from build123d import *

# Parameters (mm, degrees)
BOSS_EXTRUDE1_DEPTH             = 1
BOSS_EXTRUDE5_DEPTH             = 100
BOSS_EXTRUDE5_DEPTH_BACK        = 1
SKETCH2_W                       = 214
SKETCH2_H                       = 10
FILLET3_SIZE                    = 15
FILLET3_SIZE_2                  = 10
CUT_EXTRUDE2_DEPTH              = 229
SKETCH7_W                       = 64
SKETCH7_H                       = 10
CUT_EXTRUDE3_DEPTH              = 14
SKETCH11_R                      = 5
SKETCH11_R_2                    = 2.5
EXTRUDE_THIN4_DEPTH             = 23
EXTRUDE_THIN5_START             = -63.5
SKETCH11_2_R                    = 5
SKETCH11_2_R_2                  = 2.5
EXTRUDE_THIN5_DEPTH             = 23
EXTRUDE_THIN6_START             = -127
SKETCH11_3_R                    = 5
SKETCH11_3_R_2                  = 2.5
EXTRUDE_THIN6_DEPTH             = 23
SKETCH12_W                      = 210
SKETCH12_H                      = 6
CUT_EXTRUDE4_DEPTH              = 82
CUT_EXTRUDE5_DEPTH              = 180
SKETCH14_W                      = 83.209760426
SKETCH14_H                      = 10
BOSS_EXTRUDE6_DEPTH             = 2
SKETCH15_W                      = 1.646756057
SKETCH15_H                      = 0.570147936
SKETCH15_W_2                    = 1.681570062
SKETCH15_H_2                    = 0.299582691
CUT_EXTRUDE6_DEPTH              = 182
SKETCH16_W                      = 150
SKETCH16_H                      = 42
CUT_EXTRUDE7_DEPTH              = 182
BOSS_EXTRUDE7_REACH             = 107.948
BOSS_EXTRUDE7_END_RADIUS        = 5
BOSS_EXTRUDE7_START             = -10
SKETCH17_W                      = 23
SKETCH17_H                      = 5
BOSS_EXTRUDE7_DIRECTION_2_DEPTH = 1
FILLET5_SIZE                    = 10
FILLET5_SIZE_2                  = 1


with BuildPart() as part:
    # Sketch1 → Boss-Extrude1 (new body)
    with BuildSketch(Plane.XY):
        Polygon((75, 50), (75, -50), (-75, -30), (-75, 30), align=None)
    extrude(amount=BOSS_EXTRUDE1_DEPTH)

    # Sketch2 → Boss-Extrude5 (add, two sides: drawn at the far end of the back side and taken through both)
    with BuildSketch(Plane.XY.offset(1).offset(-BOSS_EXTRUDE5_DEPTH_BACK)):
        with Locations((32, 0)):
            Rectangle(SKETCH2_W, SKETCH2_H)
    extrude(amount=BOSS_EXTRUDE5_DEPTH + BOSS_EXTRUDE5_DEPTH_BACK)

    # Fillet3
    # an asymmetric fillet: 15, 10 mm, written as the material it adds along each edge
    with BuildSketch(Plane(origin=(75, -5, 1), x_dir=(0, 0, 1), z_dir=(-1, 0, 0))) as fillet3_piece_1:
        with BuildLine():
            Bezier((FILLET3_SIZE, 0), (0, 0), (0, -FILLET3_SIZE_2), weights=[1, 0.707106781, 1])
            Line((0, -FILLET3_SIZE_2), (0, 0))
            Line((0, 0), (FILLET3_SIZE, 0))
        make_face()
    extrude(amount=150)
    with BuildSketch(Plane(origin=(-75, 5, 1), x_dir=(0, 1, 0), z_dir=(1, 0, 0))) as fillet3_piece_2:
        with BuildLine():
            Bezier((FILLET3_SIZE_2, 0), (0, 0), (0, FILLET3_SIZE), weights=[1, 0.707106781, 1])
            Line((0, FILLET3_SIZE), (0, 0))
            Line((0, 0), (FILLET3_SIZE_2, 0))
        make_face()
    extrude(amount=150)

    # Sketch6 → Cut-Extrude2 (cut)
    with BuildSketch(Plane.ZY.offset(75)):
        with BuildLine():
            Line((9.5, 6.986773712), (9.5, 4.330127019))
            ThreePointArc((9.5, 4.330127019), (7, 0), (9.5, -4.330127019))
            Line((9.5, -4.330127019), (9.5, -7.297871365))
            Line((9.5, -7.297871365), (14.5, -7.297871365))
            Line((14.5, -7.297871365), (14.5, -4.330127019))
            ThreePointArc((14.5, -4.330127019), (17, 0), (14.5, 4.330127019))
            Line((14.5, 4.330127019), (14.5, 6.986773712))
            Line((14.5, 6.986773712), (9.5, 6.986773712))
        make_face()
    extrude(amount=-CUT_EXTRUDE2_DEPTH, mode=Mode.SUBTRACT)


with BuildPart() as cut_extrude2_piece_1:
    # of the separate pieces the step leaves, piece 1, a body of its own (cut_extrude2_pieces)
    add(part.part.solids().sort_by_distance((-75, 5.050125629, 14.5))[0])

    # Sketch11 → Extrude-Thin4 (add)
    with BuildSketch(Plane.ZY.offset(75)):
        with Locations((12, 0)):
            Circle(SKETCH11_R)
        with Locations((12, 0)):
            Circle(SKETCH11_R_2, mode=Mode.SUBTRACT)
    extrude(amount=-EXTRUDE_THIN4_DEPTH)

    # Sketch11<2> → Extrude-Thin5 (add)
    with BuildSketch(Plane.ZY.offset(75).offset(EXTRUDE_THIN5_START)):
        with Locations((12, 0)):
            Circle(SKETCH11_2_R)
        with Locations((12, 0)):
            Circle(SKETCH11_2_R_2, mode=Mode.SUBTRACT)
    extrude(amount=-EXTRUDE_THIN5_DEPTH)

    # Sketch11<3> → Extrude-Thin6 (add)
    with BuildSketch(Plane.ZY.offset(75).offset(EXTRUDE_THIN6_START)):
        with Locations((12, 0)):
            Circle(SKETCH11_3_R)
        with Locations((12, 0)):
            Circle(SKETCH11_3_R_2, mode=Mode.SUBTRACT)
    extrude(amount=-EXTRUDE_THIN6_DEPTH)

    # Sketch12 → Cut-Extrude4 (cut)
    with BuildSketch(Plane.XY.offset(101)):
        with Locations((32, 0)):
            Rectangle(SKETCH12_W, SKETCH12_H)
    extrude(amount=-CUT_EXTRUDE4_DEPTH, mode=Mode.SUBTRACT)

    # Sketch13 → Cut-Extrude5 (cut)
    with BuildSketch(Plane.XY):
        Polygon((75, 14.806657355), (75, -17.321011219), (144.128197091, -17.321011219), (144.128197091, 20.114706945), (75, 18.438480759), align=None)
    extrude(amount=CUT_EXTRUDE5_DEPTH, mode=Mode.SUBTRACT)

    # Sketch14 → Boss-Extrude6 (add)
    with BuildSketch(Plane(origin=(75, 0, 0), x_dir=(0, 0, -1), z_dir=(1, 0, 0))):
        with Locations((-59.395119787, 0)):
            Rectangle(SKETCH14_W, SKETCH14_H)
    extrude(amount=-BOSS_EXTRUDE6_DEPTH)

    # Sketch15 → Cut-Extrude6 (cut)
    with BuildSketch(Plane(origin=(75, 0, 0), x_dir=(0, 0, -1), z_dir=(1, 0, 0))):
        with Locations((-15.176621972, 5.285073968)):
            Rectangle(SKETCH15_W, SKETCH15_H)
        with Locations((-15.159214969, -5.149791346)):
            Rectangle(SKETCH15_W_2, SKETCH15_H_2)
    extrude(amount=-CUT_EXTRUDE6_DEPTH, mode=Mode.SUBTRACT)

    # Sketch16 → Cut-Extrude7 (cut)
    with BuildSketch(Plane(origin=(0, -5, 0), x_dir=(-1, 0, 0), z_dir=(0, -1, 0))):
        with Locations((0, -80)):
            Rectangle(SKETCH16_W, SKETCH16_H)
    extrude(amount=-CUT_EXTRUDE7_DEPTH, mode=Mode.SUBTRACT)

    # Boss-Extrude7: up to this cylinder (the profile starts outside it)
    boss_extrude7_end = Plane(origin=(0, 0, 12), z_dir=(-1, 0, 0)) * Cylinder(BOSS_EXTRUDE7_END_RADIUS, 353.896, mode=Mode.PRIVATE)
    # Sketch17 → Boss-Extrude7 (add, up to the surface)
    with BuildSketch(Plane.XZ.offset(5).offset(BOSS_EXTRUDE7_START), mode=Mode.PRIVATE) as boss_extrude7_sk1:
        with Locations((63.5, 12)):
            Rectangle(SKETCH17_W, SKETCH17_H)
    boss_extrude7_tool1 = extrude(boss_extrude7_sk1.sketch, amount=BOSS_EXTRUDE7_REACH, mode=Mode.PRIVATE) - boss_extrude7_end
    add(boss_extrude7_tool1.solids().sort_by_distance((63.5, 5, 12))[0])
    add(boss_extrude7_tool1.solids().sort_by_distance((63.5, 5, 12))[1])
    # Sketch17 → Boss-Extrude7 (add, up to the surface)
    with BuildSketch(Plane.XZ.offset(5).offset(BOSS_EXTRUDE7_START), mode=Mode.PRIVATE) as boss_extrude7_sk2:
        with Locations((0, 12)):
            Rectangle(SKETCH17_W, SKETCH17_H)
    boss_extrude7_tool2 = extrude(boss_extrude7_sk2.sketch, amount=BOSS_EXTRUDE7_REACH, mode=Mode.PRIVATE) - boss_extrude7_end
    add(boss_extrude7_tool2.solids().sort_by_distance((0, 5, 12))[0])
    add(boss_extrude7_tool2.solids().sort_by_distance((0, 5, 12))[1])
    # Sketch17 → Boss-Extrude7 (add, up to the surface)
    with BuildSketch(Plane.XZ.offset(5).offset(BOSS_EXTRUDE7_START), mode=Mode.PRIVATE) as boss_extrude7_sk3:
        with Locations((-63.5, 12)):
            Rectangle(SKETCH17_W, SKETCH17_H)
    boss_extrude7_tool3 = extrude(boss_extrude7_sk3.sketch, amount=BOSS_EXTRUDE7_REACH, mode=Mode.PRIVATE) - boss_extrude7_end
    add(boss_extrude7_tool3.solids().sort_by_distance((-63.5, 5, 12))[0])
    add(boss_extrude7_tool3.solids().sort_by_distance((-63.5, 5, 12))[1])

    # Sketch17 → Boss-Extrude7 direction 2 (add)
    with BuildSketch(Plane.XZ.offset(5).offset(BOSS_EXTRUDE7_START)):
        with Locations((63.5, 12)):
            Rectangle(SKETCH17_W, SKETCH17_H)
        with Locations((0, 12)):
            Rectangle(SKETCH17_W, SKETCH17_H)
        with Locations((-63.5, 12)):
            Rectangle(SKETCH17_W, SKETCH17_H)
    extrude(amount=-BOSS_EXTRUDE7_DIRECTION_2_DEPTH)

    # Fillet5
    # an asymmetric fillet: 10, 1 mm, written as the material it takes off along each edge
    with BuildSketch(Plane(origin=(-100, 6, 14.5), x_dir=(0, 0, -1), z_dir=(1, 0, 0)), Plane(origin=(-36.5, 6, 14.5), x_dir=(0, 0, -1), z_dir=(1, 0, 0)), Plane(origin=(27, 6, 14.5), x_dir=(0, 0, -1), z_dir=(1, 0, 0))) as fillet5_piece_1:
        with BuildLine():
            Bezier((FILLET5_SIZE, 0), (0, 0), (0, -FILLET5_SIZE_2), weights=[1, 0.707106781, 1])
            Line((0, -FILLET5_SIZE_2), (0, 0))
            Line((0, 0), (FILLET5_SIZE, 0))
        make_face()
    extrude(amount=73, mode=Mode.SUBTRACT)


with BuildPart() as cut_extrude2_piece_2:
    # of the separate pieces the step leaves, piece 2, a body of its own (cut_extrude2_pieces)
    add(part.part.solids().sort_by_distance((-75, 15, 1))[0])

    # Sketch7 → Cut-Extrude3 (cut)
    with BuildSketch(Plane(origin=(0, 0, 0), x_dir=(-1, 0, 0), z_dir=(0, 0, -1))):
        with Locations((-107, 0)):
            Rectangle(SKETCH7_W, SKETCH7_H)
    extrude(amount=-CUT_EXTRUDE3_DEPTH, mode=Mode.SUBTRACT)


solid = cut_extrude2_piece_1.part
Verification items for the finished model (mm, model axes). A direction names the side the tool comes from. Give positions to 0.01 mm unless a question says otherwise; leave off trailing zeros. Loops run counter-clockwise (first coordinate to the right, second up) from the corner with the lowest first, then second, coordinate; pieces in that order, holes last.
1. Go/stop test with flat-tipped pins: P1, Ø8, axis at x = 43.5, z = 21, coming from the +Y side; P2, Ø0.8, axis at x = 1.5, y = 5, coming from the -Z side; P3, Ø3, axis at x = -20.5, y = 0, coming from the +Z side; P4, Ø4, axis at y = 0, z = 12, coming from the +X side. Record where each tip stops, or that it passes through.
Derived:
P1: stops at y = 5
P2: stops at z = 9.5
P3: stops at z = 19
P4: passes through
2. Cross-section at C-C on z = 12. Count the separate pieces of the cut face and the enclosed holes in it, and give its area (3 significant figures).
Derived:
separate pieces: 6
enclosed holes: 0
area: 391 mm2
3. Tool access check on faces 5 (the flat face through (-1, 5, 37)), 6 (the flat face through (-1, 0, 19)), 7 (the flat face through (-11.5, 3, 12)). Record the directions out of +Z, -Z, +X, -X, +Y, -Y that give a thin tool (end or side, any length) a straight path to the whole face; none if there is none.
Derived:
face 5: +Z, +X, -X, +Y
face 6: +Z
face 7: -Z
4. Material ranges on probe 1 along X at (y, z) = (-3.25, 13); probe 2 along X at (y, z) = (-0.25, 54); probe 3 along Y at (x, z) = (27, 44), recorded low to high.
Derived:
probe 1: x = -75 to -52, -11.5 to 11.5, 52 to 75
probe 2: x = -75 to -73, 73 to 75
probe 3: y = -5 to -3, 3 to 5
5. Cross-section at B-B on z = 45. Record the cut outline in (x, y).
Derived:
outline: (-75, -5) - (75, -5) - (75, 5) - (-75, 5) - close; hole (-73, -3) - (73, -3) - (73, 3) - (-73, 3) - close
6. Cross-section at A-A on y = 0. Record the cut outline in (x, z), and give its area (3 significant figures).
Derived:
outline: (-75, 7) - (-52, 7) - (-52, 9.5) - (-75, 9.5) - close; (-75, 14.5) - (-52, 14.5) - (-52, 17) - (-11.5, 17) - (-11.5, 14.5) - (11.5, 14.5) - (11.5, 17) - (52, 17) - (52, 14.5) - (75, 14.5) - (75, 59) - (73, 59) - (73, 19) - (-73, 19) - (-73, 59) - (-75, 59) - close; (-11.5, 7) - (11.5, 7) - (11.5, 9.5) - (-11.5, 9.5) - close; (52, 7) - (75, 7) - (75, 9.5) - (52, 9.5) - close
area: 805 mm2
7. Release check for a two-part mould opening along Z. For faces 1 (the cylindrical face through (-0.2, 0.1, 9.5)), 2 (the flat face through (-1, -3, 39)), 3 (the cylindrical face through (-63.7, 0.1, 9.5)), 4 (the cylindrical face through (31, 0, 17)) record: +Z half, -Z half, draft (parallel to the pull), parting line (faces both ways), or undercut.
Derived:
face 1: undercut
face 2: draft
face 3: undercut
face 4: -Z half
